```python
from build123d import *

# Parameters (mm, degrees)
F1_DEPTH = 3
F2_R     = 23.9895203097
F3_R     = 8.8655957544
F4_R     = 13.3788231565


with BuildPart() as f1:
    # F0 (on Right) → F1 (new body)
    with BuildSketch(Plane.YZ):
        with BuildLine():
            ThreePointArc((21.4366063053, 255.0530908526), (21.8586977965, 257.5105561581), (22, 260))
            ThreePointArc((22, 260), (2.4894438419, 281.8586977965), (-21.4366063053, 264.9469091474))
            ThreePointArc((-21.4366063053, 264.9469091474), (-4.9469091474, 238.5633936947), (21.4366063053, 255.0530908526))
        make_face()
        with BuildLine():
            ThreePointArc((21.4366063053, 255.0530908526), (-4.9469091474, 238.5633936947), (-21.4366063053, 264.9469091474))
            Line((-21.4366063053, 264.9469091474), (-51.4366063053, 134.9469091474))
            ThreePointArc((-51.4366063053, 134.9469091474), (-28.2998058213, 151.9342047897), (-8.0571283842, 131.5844195316))
            Line((-8.0571283842, 131.5844195316), (-7.8185739981, 128.2806428715))
            Line((-7.8185739981, 128.2806428715), (21.4366063053, 255.0530908526))
        make_face()
        with BuildLine():
            ThreePointArc((-8.0571283842, 131.5844195316), (-28.2998058213, 151.9342047897), (-51.4366063053, 134.9469091474))
            ThreePointArc((-51.4366063053, 134.9469091474), (-51.9342047897, 131.7001941787), (-51.9428716158, 128.4155804684))
            ThreePointArc((-51.9428716158, 128.4155804684), (-31.7001941787, 108.0657952103), (-8.5633936947, 125.0530908526))
            ThreePointArc((-8.5633936947, 125.0530908526), (-8.1413022035, 127.5105561581), (-8, 130))
            ThreePointArc((-8, 130), (-8.0142867349, 130.7927245588), (-8.0571283842, 131.5844195316))
        make_face()
        with BuildLine():
            Line((-8.5633936947, 125.0530908526), (-7.8185739981, 128.2806428715))
            Line((-7.8185739981, 128.2806428715), (-8.0571283842, 131.5844195316))
            ThreePointArc((-8.0571283842, 131.5844195316), (-8.0142867349, 130.7927245588), (-8, 130))
            ThreePointArc((-8, 130), (-8.1413022035, 127.5105561581), (-8.5633936947, 125.0530908526))
        make_face()
        with BuildLine():
            Line((0, 20), (-7.8185739981, 128.2806428715))
            Line((-7.8185739981, 128.2806428715), (-8.5633936947, 125.0530908526))
            ThreePointArc((-8.5633936947, 125.0530908526), (-31.7001941787, 108.0657952103), (-51.9428716158, 128.4155804684))
            Line((-51.9428716158, 128.4155804684), (-44.1145542365, 20))
            Line((-44.1145542365, 20), (0, 20))
        make_face()
        Polygon((0, 0), (0, 20), (-44.1145542365, 20), (-100, 20), (-100, 0), align=None)
    extrude(amount=F1_DEPTH)

    # F2
    f2_edges = [f1.edges().sort_by_distance(p)[0] for p in [
        (1.5, -44.114554, 20),
    ]]
    fillet(f2_edges, radius=F2_R)

    # F3
    f3_edges = [f1.edges().sort_by_distance(p)[0] for p in [
        (1.5, -100, 20),
        (1.5, -100, 0),
    ]]
    fillet(f3_edges, radius=F3_R)

    # F4
    f4_edges = [f1.edges().sort_by_distance(p)[0] for p in [
        (1.5, 0, 0),
    ]]
    fillet(f4_edges, radius=F4_R)


solid = f1.part
```
CAD build for the part. Positions are in the model's coordinates, mm. A direction names the side the tool comes from. Give positions to 0.01 mm unless a question says otherwise; leave off trailing zeros. Loops run counter-clockwise (first coordinate to the right, second up) from the corner with the lowest first, then second, coordinate; pieces in that order, holes last. Notation, with made-up numbers: (7.25, -8.5) -> (23.25, -8.5) arc R8 cw to (23.25, 2.5) -> close; hole circle Ø8 at (42, 56.5). An arc over 180 degrees is marked (long way). Use a Markdown table: item, result.
1. Mould opens along Z. For faces 4 (the flat face through (1.479, -3.855, 73.382)), 5 (the flat face through (1.479, -36.227, 200.857)), 6 (the cylindrical face through (1.521, -97.472, 2.666)) say: pulls with the +Z half, pulls with the -Z half, needs draft (parallel to the pull), parting line crosses it, or undercut.
Check result:
| item | result |
|---|---|
| face 4 | undercut |
| face 5 | pulls with the +Z half |
| face 6 | pulls with the -Z half |
2. Slice it at A-A (x = 1.35). List the corners of the cut face in (y, z), plus the area to 3 significant figures.
Check result:
| item | result |
|---|---|
| outline | (-100, 8.87) arc R8.87 ccw to (-91.13, 0) -> (-13.38, 0) arc R13.38 ccw to (0, 13.38) -> (0, 20) -> (-7.82, 128.28) -> (21.44, 255.05) arc R22 ccw to (-21.44, 264.95) -> (-51.44, 134.95) arc R22 ccw to (-51.94, 128.42) -> (-45.97, 45.72) arc R23.99 cw to (-69.9, 20) -> (-91.13, 20) arc R8.87 ccw to (-100, 11.13) -> close |
| area | 13,600 mm^2 |
3. Which spindle directions (+Z, -Z, +X, -X, +Y, -Y) get a long thin tool onto all of the face, cutting with end or side? Do faces 1 (the flat face through (1.479, 6.604, 190.779)), 2 (the cylindrical face through (1.52, -52.15, 27.85)), 3 (the flat face through (3, -26, 143)). Say none if no direction does.
Check result:
| item | result |
|---|---|
| face 1 | +X, -X, +Y |
| face 2 | +X, -X, -Y |
| face 3 | +Z, -Z, +X, +Y, -Y |
4. Flat gauge pins, fed straight in: pin 1 (0.9 mm diameter, centred on x = 2, y = -80, fed in from +Z); pin 2 (0.9 mm diameter, centred on x = 1, z = 15.5, fed in from +Y); pin 3 (1.5 mm diameter, centred on x = 1, z = 95, fed in from +Y). Where does each tip first touch, or does it go through?
Check result:
| item | result |
|---|---|
| pin 1 | stops at z = 20 |
| pin 2 | stops at y = 0 |
| pin 3 | stops at y = -5.36 |
5. Wall check: L1, parallel to Z at x = 0.3, y = -83; L2, parallel to Y at x = 0.45, z = 221; L3, parallel to Y at x = 1, z = 83. Give the ranges that are in metal, low to high. Write a range as [from, to].
Check result:
| item | result |
|---|---|
| L1 | z = [0, 20] |
| L2 | y = [-31.58, 13.58] |
| L3 | y = [-48.66, -4.55] |
6. Slice it at B-B (y = -73). List the corners of the cut face in (x, z).
Check result:
| item | result |
|---|---|
| outline | (0, 0) -> (3, 0) -> (3, 20) -> (0, 20) -> close |
7. Slice it at C-C (z = 201). List the corners of the cut face in (x, y).
Check result:
| item | result |
|---|---|
| outline | (0, -36.19) -> (3, -36.19) -> (3, 8.96) -> (0, 8.96) -> close |
